from build123d import *

# Parameters (mm, degrees)
EXTRUDE_1_DEPTH          = 10
FILLET_1_R               = 5
EXTRUDE_START            = 47
SKETCH_6_R               = 2
EXTRUDE_2_DEPTH          = 8
EXTRUDE_START_2          = -39
SKETCH_6_2_R             = 2
EXTRUDE_3_DEPTH          = 8
CUT_EXTRUDE_4_DEPTH      = 70.34695379
CUT_EXTRUDE_4_DEPTH_BACK = 70.34695379
SKETCH_7_R               = 2
CHAMFER_1_SIZE           = 2
CHAMFER_2_SIZE           = 2


with BuildPart() as part:
    # 草图1 → 凸台-拉伸1 (new body)
    with BuildSketch(Plane(origin=(0, 0, 0), x_dir=(1, 0, 0), z_dir=(0, 1, 0))):
        Polygon((-4, -50), (-10, -50), (-10, -17), (-4, -17), (-4, -8), (-47, -8), (-47, 0), (47, 0), (47, -8), (4, -8), (4, -17), (10, -17), (10, -50), (4, -50), (4, -25), (-4, -25), align=None)
    extrude(amount=EXTRUDE_1_DEPTH)

    # 圆角1
    fillet_1_edges = [part.edges().sort_by_distance(p)[0] for p in [
        (-7, 0, 50),
        (-7, 10, 50),
        (7, 10, 50),
        (7, 0, 50),
    ]]
    fillet(fillet_1_edges, radius=FILLET_1_R - 0.0001)  # a hair under: the kernel refuses the full size

    # 草图6 → 凸台-拉伸2 (add)
    with BuildSketch(Plane(origin=(0, 0, 0), x_dir=(0, 0, -1), z_dir=(1, 0, 0)).offset(EXTRUDE_START)):
        with BuildLine():
            Line((0.868240888, 9.924038765), (20.564395949, 6.451075212))
            ThreePointArc((20.564395949, 6.451075212), (24.620193825, 0.658795558), (18.827914172, -3.397002318))
            Line((18.827914172, -3.397002318), (-0.868240888, 0.075961235))
            ThreePointArc((-0.868240888, 0.075961235), (-4.924038765, 5.868240888), (0.868240888, 9.924038765))
        make_face()
        with Locations(Location((19.69615506, 1.527036447, 0), (0, 0, 180))):
            Circle(SKETCH_6_R, mode=Mode.SUBTRACT)
    extrude(amount=-EXTRUDE_2_DEPTH)

    # 草图6<2> → 凸台-拉伸3 (add)
    with BuildSketch(Plane(origin=(0, 0, 0), x_dir=(0, 0, -1), z_dir=(1, 0, 0)).offset(EXTRUDE_START_2)):
        with BuildLine():
            Line((0.868240888, 9.924038765), (20.564395949, 6.451075212))
            ThreePointArc((20.564395949, 6.451075212), (24.620193825, 0.658795558), (18.827914172, -3.397002318))
            Line((18.827914172, -3.397002318), (-0.868240888, 0.075961235))
            ThreePointArc((-0.868240888, 0.075961235), (-4.924038765, 5.868240888), (0.868240888, 9.924038765))
        make_face()
        with Locations(Location((19.69615506, 1.527036447, 0), (0, 0, 180))):
            Circle(SKETCH_6_2_R, mode=Mode.SUBTRACT)
    extrude(amount=-EXTRUDE_3_DEPTH)

    # 草图7 → 切除-拉伸4 (cut, two sides: drawn at the far end of the back side and taken through both)
    with BuildSketch(Plane(origin=(0, 0, 0), x_dir=(0, 0, -1), z_dir=(1, 0, 0)).offset(-CUT_EXTRUDE_4_DEPTH_BACK)):
        with Locations((-45, 5)):
            Circle(SKETCH_7_R)
    extrude(amount=CUT_EXTRUDE_4_DEPTH + CUT_EXTRUDE_4_DEPTH_BACK, mode=Mode.SUBTRACT)

    # 倒角1
    chamfer_1_edges = [part.edges().sort_by_distance(p)[0] for p in [
        (0, 0, 25),
        (0, 10, 25),
    ]]
    chamfer(chamfer_1_edges, length=CHAMFER_1_SIZE)

    # 倒角2
    chamfer_2_edges = [part.edges().sort_by_distance(p)[0] for p in [
        (10, 5, 17),
        (-10, 5, 17),
    ]]
    chamfer(chamfer_2_edges, length=CHAMFER_2_SIZE)


solid = part.part
Can you work these out from the model? Positions are in its coordinate system, mm. A direction names the side the tool comes from. Coordinates: 2 decimals unless noted, no trailing zeros. Loops run counter-clockwise (first coordinate to the right, second up) from the corner with the lowest first, then second, coordinate; pieces in that order, holes last. Notation, with made-up numbers: (-16.5, 41.5) - (18.5, 41.5) arc R35 cw to (18.5, 77.5) - close; hole circle Ø9 at (20, 46.25). An arc over 180 degrees is marked (long way). Answer as a JSON object with one key per item and string values. Group by question number.
Item 1: If we section it at B-B (z = 1.5): List the corners of the cut face in (x, y) for me.
Item 2: If we section it at C-C (z = 13): List the corners of the cut face in (x, y) for me.
Item 3: On a 3-axis mill with a long thin cutter (end or side, diameter ignored), from which of +Z, -Z, +X, -X, +Y, -Y can I reach the whole of each face in a straight line? I mean faces 5 (the face through (39, 3, -12)), 6 (the face through (6, 5, 17)), 7 (the face through (-6, 5, 17)), 8 (the face through (-47, 3, -9)), 9 (the face through (47, 3, -9)). Say none if no direction works.
Item 4: If we mould it in two halves opening along X, with no side actions, what happens to faces 1 (the face through (-10, 5, 35)), 2 (the face through (0, 5, 25)), 3 (the face through (0, 10, 11)), 4 (the face through (-4, 5, 36))? For each: released by +X, released by -X, zero draft, split by the parting line, or undercut.
Item 5: If we section it at A-A (x = 6.5): State how many separate pieces and enclosed holes the cut face has, plus the area to 3 significant figures.
Item 6: If I drill on L1, parallel to X at y = 6, z = -10.5; L2, parallel to X at y = 6.5, z = 43; L3, parallel to Y at x = -5.65, z = 45, over which ranges is the centre line in solid material (lowest first)? Write a range as from..to.
Item 7: For pin 1 (2 mm diameter, centred on x = 6, y = 4.5, fed in from -Z); pin 2 (3 mm diameter, centred on y = 5, z = 36, fed in from +X); pin 3 (8 mm diameter, centred on y = 5, z = 28, fed in from -X), each with a flat end and sliding along its axis, tell me the tip position at first contact or that it passes through.
Returned:
{
 "1": {"outline": "(-47, 0) - (47, 0) - (47, 10) - (-47, 10) - close"},
 "2": {"outline": "(-4, 0) - (4, 0) - (4, 10) - (-4, 10) - close"},
 "3": {"face 5": "-Z, +Y, -Y", "face 6": "+X, +Y, -Y", "face 7": "-X, +Y, -Y", "face 8": "+Z, -Z, -X, +Y, -Y", "face 9": "+Z, -Z, +X, +Y, -Y"},
 "4": {"face 1": "released by -X", "face 2": "undercut", "face 3": "zero draft", "face 4": "undercut"},
 "5": {"separate pieces": "2", "enclosed holes": "1", "area": "387 mm²"},
 "6": {"L1": "x = -47..-39, 39..47", "L2": "x = -10..-4, 4..10", "L3": "y = 0..3, 7..10"},
 "7": {"pin 1": "stops at z = 0", "pin 2": "stops at x = 10", "pin 3": "stops at x = -10"}
}
